Check sheet for the modelled part. Datum: model origin and axes. Units: mm. A direction names the side the tool comes from. Coordinates: 2 decimals unless noted, no trailing zeros. Loops run counter-clockwise (first coordinate to the right, second up) from the corner with the lowest first, then second, coordinate; pieces in that order, holes last. Notation, with made-up numbers: (7, 65.25) - (23, 65.25) arc R28 ccw to (23, 95.25) - close; hole circle Ø9 at (-25, 27). An arc over 180 degrees is marked (long way). Use a Markdown table: item, result. Add a question column.
1) Sectioned sample at B-B, the plane y = 13.5. Enter the section's corners in (x, z).
2) Go/stop test with flat-tipped pins: P1, Ø2, axis at x = 17, y = 28, coming from the -Z side; P2, Ø16, axis at x = -30, z = -10, coming from the -Y side; P3, Ø11.5, axis at x = 30, z = -10, coming from the +Y side; P4, Ø5, axis at x = 13.5, y = 30.5, coming from the +Z side. Record where each tip stops, or that it passes through.
3) Sectioned sample at A-A, the plane z = -80. Enter the section's corners in (x, y), then the cut area to 3 significant figures.
4) Thickness scan on line 1 (X direction, y = 15.75, z = -10); line 2 (Z direction, x = 29, y = 13); line 3 (Z direction, x = 27.5, y = 2). Record the ranges inside material, lowest first.
5) Sectioned sample at C-C, the plane x = 30. State how many separate pieces and enclosed holes the cut face has, then the cut area to 3 significant figures.
6) Tool access check on faces 4 (the flat face through (30, 0, -44)), 5 (the flat face through (20, 3, -44)), 6 (the flat face through (-8, 25, -18)). Record the directions out of +Z, -Z, +X, -X, +Y, -Y that give a thin tool (end or side, any length) a straight path to the whole face; none if there is none.
7) Draft check along Z on faces 1 (the flat face through (-1, 13, -90)), 2 (the cylindrical face through (-31.915, 12.675, -75.381)), 3 (the flat face through (9, 25, -71)). Enter one of: pulls with the +Z half, pulls with the -Z half, needs draft (parallel to the pull), parting line crosses it, or undercut.
from build123d import *

# Parameters (mm, degrees)
SALIENTE_EXTRUIR1_DEPTH = 90
CORTAR_EXTRUIR1_REACH   = 103.612
CROQUIS13_R             = 5


with BuildPart() as part:
    # Croquis1 → Saliente-Extruir1 (new body)
    with BuildSketch(Plane.XY):
        Polygon((-20, 0), (-20, 6), (20, 6), (20, 0), (40, 0), (40, 25), (-40, 25), (-40, 0), align=None)
    extrude(amount=-SALIENTE_EXTRUIR1_DEPTH)

    # Croquis7 → Recubrir5 section 0
    with BuildSketch(Plane.ZY.offset(40)):
        with BuildLine():
            Line((-72.5, 25), (-47.5, 25))
            ThreePointArc((-47.5, 25), (-60, 37.5), (-72.5, 25))
        make_face()
    # Croquis4 → Recubrir5 section 1
    with BuildSketch(Plane(origin=(40, 0, 0), x_dir=(0, 0, -1), z_dir=(1, 0, 0))):
        with BuildLine():
            Line((17.5, 25), (42.5, 25))
            ThreePointArc((42.5, 25), (30, 37.5), (17.5, 25))
        make_face()
    loft()

    # Cortar-Recubrir9: read off the stored shape, not the designer's step
    # Cortar-Recubrir9: loft between two sections, ruled curve by curve
    cortar_recubrir9_from = [
        Edge.make_bspline([(40, 32.499166066, -30.111840594), (40, 32.489846016, -30.7367711), (40, 32.403311627, -31.442559169), (40, 32.050170272, -32.589420619), (40, 31.894761884, -32.985674675), (40, 31.488867377, -33.787689912), (40, 31.23815997, -34.193490215), (40, 30.626297022, -34.984454015), (40, 30.264857287, -35.369499204), (40, 29.428532809, -36.077692088), (40, 28.953437789, -36.400496106), (40, 27.907235106, -36.938588098), (40, 27.33619148, -37.153384345), (40, 26.13890697, -37.438520628), (40, 25.513089911, -37.508486115), (40, 24.2632289, -37.489846016), (40, 23.639776598, -37.401249254), (40, 22.451527572, -37.08053575), (40, 21.887143317, -36.84880603), (40, 20.857452279, -36.279754704), (40, 20.392194841, -35.942926515), (40, 19.577361218, -35.210108693), (40, 19.227564602, -34.814456311), (40, 18.63956098, -34.005598017), (40, 18.40106638, -33.592501883), (40, 18.019269161, -32.778739219), (40, 17.875746519, -32.378026983), (40, 17.556962594, -31.221144617), (40, 17.491513885, -30.513089911), (40, 17.510153984, -29.2632289), (40, 17.596688373, -28.557440831), (40, 17.949829728, -27.410579381), (40, 18.105238116, -27.014325325), (40, 18.511132623, -26.212310088), (40, 18.76184003, -25.806509785), (40, 19.373702978, -25.015545985), (40, 19.735142713, -24.630500796), (40, 20.571467191, -23.922307912), (40, 21.046562211, -23.599503894), (40, 22.092764894, -23.061411902), (40, 22.66380852, -22.846615655), (40, 23.86109303, -22.561479372), (40, 24.486910089, -22.491513885), (40, 25.7367711, -22.510153984), (40, 26.360223402, -22.598750746), (40, 27.548472428, -22.91946425), (40, 28.112856683, -23.15119397), (40, 29.142547721, -23.720245296), (40, 29.607805159, -24.057073485), (40, 30.422638782, -24.789891307), (40, 30.772435398, -25.185543689), (40, 31.36043902, -25.994401983), (40, 31.59893362, -26.407498117), (40, 31.980730839, -27.221260781), (40, 32.124253481, -27.621973017), (40, 32.443037406, -28.778855383), (40, 32.508486115, -29.486910089), (40, 32.499166066, -30.111840594)], [0, 0, 0, 0, 0.0625, 0.0625, 0.09375, 0.09375, 0.125, 0.125, 0.15625, 0.15625, 0.1875, 0.1875, 0.21875, 0.21875, 0.25, 0.25, 0.28125, 0.28125, 0.3125, 0.3125, 0.34375, 0.34375, 0.375, 0.375, 0.40625, 0.40625, 0.4375, 0.4375, 0.5, 0.5, 0.5625, 0.5625, 0.59375, 0.59375, 0.625, 0.625, 0.65625, 0.65625, 0.6875, 0.6875, 0.71875, 0.71875, 0.75, 0.75, 0.78125, 0.78125, 0.8125, 0.8125, 0.84375, 0.84375, 0.875, 0.875, 0.90625, 0.90625, 0.9375, 0.9375, 1, 1, 1, 1], 3),
    ]
    cortar_recubrir9_to = [
        Edge.make_bspline([(-40, 32.407786034, -58.827521395), (-40, 32.505492584, -59.444836898), (-40, 32.540952669, -60.155025311), (-40, 32.389176568, -61.345388288), (-40, 32.303834333, -61.762384388), (-40, 32.041099336, -62.622005881), (-40, 31.863495239, -63.064707671), (-40, 31.395936741, -63.948669802), (-40, 31.105682099, -64.38986219), (-40, 30.4028125, -65.230665449), (-40, 29.989931581, -65.629973674), (-40, 29.051182223, -66.33908064), (-40, 28.525292772, -66.648383946), (-40, 27.394421955, -67.134104129), (-40, 26.789794107, -67.310079483), (-40, 25.555163102, -67.505492584), (-40, 24.925744385, -67.524837827), (-40, 23.700150248, -67.41209072), (-40, 23.104447414, -67.280309139), (-40, 21.992598562, -66.895763725), (-40, 21.476585556, -66.643477599), (-40, 20.548417009, -66.060829384), (-40, 20.136101969, -65.730837282), (-40, 19.418414702, -65.034471726), (-40, 19.112777895, -64.668255626), (-40, 18.597419473, -63.931788052), (-40, 18.38747326, -63.561529181), (-40, 17.875511732, -62.476220288), (-40, 17.689920517, -61.789794107), (-40, 17.494507416, -60.555163102), (-40, 17.459047331, -59.844974689), (-40, 17.610823432, -58.654611712), (-40, 17.696165667, -58.237615612), (-40, 17.958900664, -57.377994119), (-40, 18.136504761, -56.935292329), (-40, 18.604063259, -56.051330198), (-40, 18.894317901, -55.61013781), (-40, 19.5971875, -54.769334551), (-40, 20.010068419, -54.370026326), (-40, 20.948817777, -53.66091936), (-40, 21.474707228, -53.351616054), (-40, 22.605578045, -52.865895871), (-40, 23.210205893, -52.689920517), (-40, 24.444836898, -52.494507416), (-40, 25.074255615, -52.475162173), (-40, 26.299849752, -52.58790928), (-40, 26.895552586, -52.719690861), (-40, 28.007401438, -53.104236275), (-40, 28.523414444, -53.356522401), (-40, 29.451582991, -53.939170616), (-40, 29.863898031, -54.269162718), (-40, 30.581585298, -54.965528274), (-40, 30.887222105, -55.331744374), (-40, 31.402580527, -56.068211948), (-40, 31.61252674, -56.438470819), (-40, 32.124488268, -57.523779712), (-40, 32.310079483, -58.210205893), (-40, 32.407786034, -58.827521395)], [0, 0, 0, 0, 0.0625, 0.0625, 0.09375, 0.09375, 0.125, 0.125, 0.15625, 0.15625, 0.1875, 0.1875, 0.21875, 0.21875, 0.25, 0.25, 0.28125, 0.28125, 0.3125, 0.3125, 0.34375, 0.34375, 0.375, 0.375, 0.40625, 0.40625, 0.4375, 0.4375, 0.5, 0.5, 0.5625, 0.5625, 0.59375, 0.59375, 0.625, 0.625, 0.65625, 0.65625, 0.6875, 0.6875, 0.71875, 0.71875, 0.75, 0.75, 0.78125, 0.78125, 0.8125, 0.8125, 0.84375, 0.84375, 0.875, 0.875, 0.90625, 0.90625, 0.9375, 0.9375, 1, 1, 1, 1], 3),
    ]
    cortar_recubrir9 = Solid(Shell([*[Face.make_surface_from_curves(cortar_recubrir9_from[k], cortar_recubrir9_to[k]) for k in range(1)], Face(Wire(cortar_recubrir9_from)), Face(Wire(cortar_recubrir9_to))]))
    add(cortar_recubrir9, mode=Mode.SUBTRACT)

    # Croquis13 → Cortar-Extruir1 (cut, up to next)
    with BuildSketch(Plane(origin=(0, 25, 0), x_dir=(1, 0, 0), z_dir=(0, 1, 0)), mode=Mode.PRIVATE) as cortar_extruir1_sk1:
        with Locations(Location((-30, 80, 0), (0, 0, 270))):
            Circle(CROQUIS13_R)
    cortar_extruir1_tool1 = extrude(cortar_extruir1_sk1.sketch, amount=-CORTAR_EXTRUIR1_REACH, mode=Mode.PRIVATE) & part.part
    # Croquis13 → Cortar-Extruir1 (cut, up to next)
    with BuildSketch(Plane(origin=(0, 25, 0), x_dir=(1, 0, 0), z_dir=(0, 1, 0)), mode=Mode.PRIVATE) as cortar_extruir1_sk2:
        with Locations((30, 80)):
            Circle(CROQUIS13_R)
    cortar_extruir1_tool2 = extrude(cortar_extruir1_sk2.sketch, amount=-CORTAR_EXTRUIR1_REACH, mode=Mode.PRIVATE) & part.part
    # Croquis13 → Cortar-Extruir1 (cut, up to next)
    with BuildSketch(Plane(origin=(0, 25, 0), x_dir=(1, 0, 0), z_dir=(0, 1, 0)), mode=Mode.PRIVATE) as cortar_extruir1_sk3:
        with Locations(Location((30, 10, 0), (0, 0, 270))):
            Circle(CROQUIS13_R)
    cortar_extruir1_tool3 = extrude(cortar_extruir1_sk3.sketch, amount=-CORTAR_EXTRUIR1_REACH, mode=Mode.PRIVATE) & part.part
    # Croquis13 → Cortar-Extruir1 (cut, up to next)
    with BuildSketch(Plane(origin=(0, 25, 0), x_dir=(1, 0, 0), z_dir=(0, 1, 0)), mode=Mode.PRIVATE) as cortar_extruir1_sk4:
        with Locations(Location((-30, 10, 0), (0, 0, 90))):
            Circle(CROQUIS13_R)
    cortar_extruir1_tool4 = extrude(cortar_extruir1_sk4.sketch, amount=-CORTAR_EXTRUIR1_REACH, mode=Mode.PRIVATE) & part.part
    add(cortar_extruir1_tool1.solids().sort_by_distance((-30, 25, -80))[0], mode=Mode.SUBTRACT)
    add(cortar_extruir1_tool2.solids().sort_by_distance((30, 25, -80))[0], mode=Mode.SUBTRACT)
    add(cortar_extruir1_tool3.solids().sort_by_distance((30, 25, -10))[0], mode=Mode.SUBTRACT)
    add(cortar_extruir1_tool4.solids().sort_by_distance((-30, 25, -10))[0], mode=Mode.SUBTRACT)


solid = part.part
Solved:
| question | item | result |
|---|---|---|
| 1 | outline | (-40, -90) - (40, -90) - (40, 0) - (-40, 0) - close; hole circle Ø10 at (-30, -80); hole circle Ø10 at (-30, -10); hole circle Ø10 at (30, -80); hole circle Ø10 at (30, -10) |
| 2 | P1 | stops at z = -51.2 |
| 2 | P2 | stops at y = 0 |
| 2 | P3 | stops at y = 25 |
| 2 | P4 | stops at z = -27.34 |
| 3 | outline | (-40, 0) - (-35, 0) - (-35, 25) - (-40, 25) - close; (-25, 0) - (-20, 0) - (-20, 6) - (20, 6) - (20, 0) - (25, 0) - (25, 25) - (-25, 25) - close; (35, 0) - (40, 0) - (40, 25) - (35, 25) - close |
| 3 | area | 1,260 mm2 |
| 4 | line 1 | x = -40 to -35, -25 to 25, 35 to 40 |
| 4 | line 2 | z = -90 to -84.9, -75.1 to -14.9, -5.1 to 0 |
| 4 | line 3 | z = -90 to -84.33, -75.67 to -14.33, -5.67 to 0 |
| 5 | separate pieces | 3 |
| 5 | enclosed holes | 1 |
| 5 | area | 1,820 mm2 |
| 6 | face 4 | +Z, -Z, +X, -X, -Y |
| 6 | face 5 | +Z, -Z, -Y |
| 6 | face 6 | +Z, -X, +Y |
| 7 | face 1 | pulls with the -Z half |
| 7 | face 2 | undercut |
| 7 | face 3 | needs draft |
